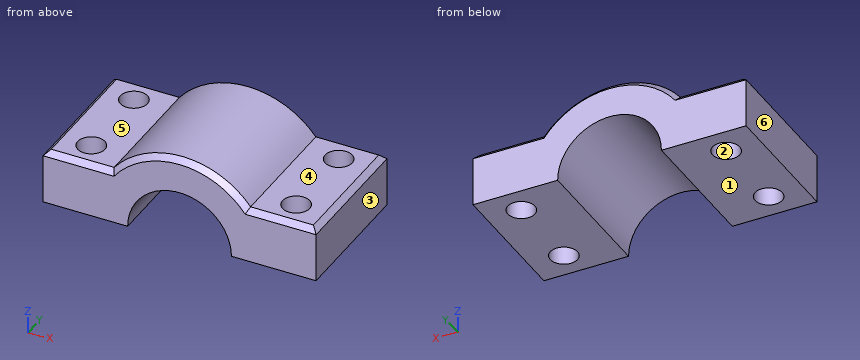
```python
from build123d import *

# Parameters (mm, degrees)
SKETCH_1_R          = 8
EXTRUDE_1_DEPTH     = 12.5
SKETCH_3_W          = 25
SKETCH_3_H          = 10
EXTRUDE_2_DEPTH     = 12.5
SKETCH_4_R          = 4.75
CUT_EXTRUDE_1_DEPTH = 20.403607912
SKETCH_5_R          = 1.25
CUT_EXTRUDE_2_DEPTH = 22.943108257
CHAMFER_1_SIZE      = 0.5
SKETCH_6_W          = 49.161013252
SKETCH_6_H          = 46.40097955
CUT_EXTRUDE_3_DEPTH = 20.403607912


with BuildPart() as part:
    # 草图1 → 凸台-拉伸1 (new body)
    with BuildSketch(Plane(origin=(0, 0, 0), x_dir=(1, 0, 0), z_dir=(0, 1, 0))):
        with Locations(Location((0, 0, 0), (0, 0, 270))):
            Circle(SKETCH_1_R)
    extrude(amount=EXTRUDE_1_DEPTH)

    # 草图3 → 凸台-拉伸2 (add)
    with BuildSketch(Plane(origin=(0, 12.5, 0), x_dir=(1, 0, 0), z_dir=(0, 1, 0))):
        Rectangle(SKETCH_3_W, SKETCH_3_H)
    extrude(amount=-EXTRUDE_2_DEPTH)

    # 草图4 → 切除-拉伸1 (cut, through all)
    with BuildSketch(Plane(origin=(0, 12.5, 0), x_dir=(1, 0, 0), z_dir=(0, 1, 0))):
        with Locations(Location((0, 0, 0), (0, 0, 270))):
            Circle(SKETCH_4_R)
    extrude(amount=-CUT_EXTRUDE_1_DEPTH, mode=Mode.SUBTRACT)

    # 草图5 → 切除-拉伸2 (cut, through all)
    with BuildSketch(Plane(origin=(0, 0, -5), x_dir=(-1, 0, 0), z_dir=(0, 0, -1))):
        with Locations((9.372498999, 2.5)):
            Circle(SKETCH_5_R)
        with Locations((9.372498999, 10)):
            Circle(SKETCH_5_R)
    cut_extrude_2 = extrude(amount=-CUT_EXTRUDE_2_DEPTH, mode=Mode.SUBTRACT)

    # 镜向1: 切除-拉伸2 across plane
    add(cut_extrude_2.mirror(Plane(origin=(0, 0, 0), x_dir=(0, 0, 1), z_dir=(1, 0, 0))), mode=Mode.SUBTRACT)

    # 倒角1
    chamfer_1_edges = [part.edges().sort_by_distance(p)[0] for p in [
        (9.372498999, 12.5, -5),
        (9.372498999, 12.5, 5),
        (9.372498999, 0, 5),
        (9.372498999, 0, -5),
        (-12.5, 6.25, -5),
        (12.5, 6.25, 5),
        (-12.5, 6.25, 5),
        (12.5, 6.25, -5),
        (-9.372498999, 12.5, 5),
        (-9.372498999, 12.5, -5),
        (-9.372498999, 0, -5),
        (-9.372498999, 0, 5),
        (0, 0, -8),
        (0, 0, 8),
        (0, 12.5, -8),
        (0, 12.5, 8),
    ]]
    chamfer(chamfer_1_edges, length=CHAMFER_1_SIZE)

    # 草图6 → 切除-拉伸3 (cut, through all)
    with BuildSketch(Plane.XY):
        Rectangle(SKETCH_6_W, SKETCH_6_H)
    extrude(amount=-CUT_EXTRUDE_3_DEPTH, mode=Mode.SUBTRACT)


solid = part.part
```
Geometry check sheet. Reference: the model listing, model coordinates, mm. Face numbers are marked on the shaded views. A direction names the side the tool comes from. Give positions to 0.01 mm unless a question says otherwise; leave off trailing zeros. Loops run counter-clockwise (first coordinate to the right, second up) from the corner with the lowest first, then second, coordinate; pieces in that order, holes last. Notation, with made-up numbers: (11, -38) - (54, -38) arc R12 cw to (54, -20) - close; hole circle Ø8 at (30.5, 69). An arc over 180 degrees is marked (long way). Use CSV: the item, a comma, the result in double quotes. Start each with the question number.
Q1. Release check for a two-part mould opening along X. For the marked faces 1, 2 and 3 record: +X half, -X half, draft (parallel to the pull), parting line (faces both ways), or undercut.
Q2. Section check D-D, the plane z = 2. Record the cut outline in (x, y), and give its area (3 significant figures).
Q3. Section check C-C, the plane x = 10. Record the cut outline in (y, z), and give its area (3 significant figures).
Q4. Section check A-A, the plane z = 3.25. Record the cut outline in (x, y), and give its area (3 significant figures).
Q5. Access from +Z, -Z, +X, -X, +Y, -Y to the whole of each face (thin tool, end or side, straight path). Record for the marked faces 4, 5 and 6.
Q6. Go/stop test with flat-tipped pins: pin 1 Ø1 at (x, y) = (-9, 10) entering from +Z; pin 2 Ø6.5 at (x, y) = (-8.5, 4) entering from +Z; pin 3 Ø1.7 at (x, y) = (9.5, 6) entering from +Z. Record where each tip stops, or that it passes through.
Q7. Section check B-B, the plane y = 10. Count the separate pieces of the cut face and the enclosed holes in it, and give its area (3 significant figures).
Q8. Scan lines: probe 1 along Y at (x, z) = (-9.5, 4); probe 2 along Y at (x, z) = (10, 3); probe 3 along X at (y, z) = (1.5, 4.25). Record each from-to range of solid material in increasing order. Write a range as from..to.
Findings below:
1,face 1,"draft"
1,face 2,"undercut"
1,face 3,"+X half"
2,outline,"(-12.5, 0) - (-4.31, 0) - (-4.31, 12.5) - (-12.5, 12.5) - close; (4.31, 0) - (12.5, 0) - (12.5, 12.5) - (4.31, 12.5) - close; hole circle Ø2.5 at (-9.37, 2.5); hole circle Ø2.5 at (-9.37, 10); hole circle Ø2.5 at (9.37, 2.5); hole circle Ø2.5 at (9.37, 10)"
2,area,"185 mm^2"
3,outline,"(0, 0) - (1.42, 0) - (1.42, 5) - (0.5, 5) - (0, 4.5) - close; (3.58, 0) - (8.92, 0) - (8.92, 5) - (3.58, 5) - close; (11.08, 0) - (12.5, 0) - (12.5, 4.5) - (12, 5) - (11.08, 5) - close"
3,area,"40.6 mm^2"
4,outline,"(-12.5, 0) - (-3.46, 0) - (-3.46, 12.5) - (-12.5, 12.5) - close; (3.46, 0) - (12.5, 0) - (12.5, 12.5) - (3.46, 12.5) - close; hole circle Ø2.5 at (-9.37, 2.5); hole circle Ø2.5 at (-9.37, 10); hole circle Ø2.5 at (9.37, 2.5); hole circle Ø2.5 at (9.37, 10)"
4,area,"206 mm^2"
5,face 4,"+Z, +X, +Y, -Y"
5,face 5,"+Z, -X, +Y, -Y"
5,face 6,"+Z, -Z, -X, +Y, -Y"
6,pin 1,"passes through"
6,pin 2,"stops at z = 6.04"
6,pin 3,"stops at z = 5"
7,separate pieces,"3"
7,enclosed holes,"0"
7,area,"90.4 mm^2"
8,probe 1,"y = 0..1.26, 3.74..8.76, 11.24..12.5"
8,probe 2,"y = 0..1.42, 3.58..8.92, 11.08..12.5"
8,probe 3,"x = -12.5..-10.12, -8.62..-2.12, 2.12..8.62, 10.12..12.5"
